Design review of the part built by this model. Coordinates are the model's own, in mm. A direction names the side the tool comes from. Coordinates: 2 decimals unless noted, no trailing zeros. Loops run counter-clockwise (first coordinate to the right, second up) from the corner with the lowest first, then second, coordinate; pieces in that order, holes last. Notation, with made-up numbers: (10.25, 37) -> (34.25, 37) arc R31 ccw to (34.25, 76) -> close; hole circle Ø1 at (26, 66.25). An arc over 180 degrees is marked (long way). One line per item, written item: value. Start each with the question number.
1. Add section B-B on y = -4. Write out the cut boundary in (x, z), plus the area to 3 significant figures.
2. Add section C-C on x = 0.25. Write out the cut boundary in (y, z).
3. Add section A-A on z = 5. Write out the cut boundary in (x, y), plus the area to 3 significant figures.
4. Insertion check: pin 1 (2 mm diameter, centred on x = -2, y = -12, fed in from -Z); pin 2 (2 mm diameter, centred on x = -18.5, y = -7.5, fed in from +Z); pin 3 (3 mm diameter, centred on x = -6.15, y = -8, fed in from +Z). Each pin has a flat end and moves straight along its axis. Give the tip position at first contact, or say it passes through.
5. Machinability: for faces 1 (the flat face through (-12, -8, -3.642)), 2 (the cylindrical face through (-4.49, -7.31, 0.8)), 3 (the cylindrical face through (-1.1, -10.3, 7.3)), which of the approach directions +Z, -Z, +X, -X, +Y, -Y give a long, thin tool a straight path to every point of the face, cutting with its end or side? Answer none if there is none.
6. For probe 1 along Y at (x, z) = (-6, 5); probe 2 along Y at (x, z) = (0, 4.25); probe 3 along Y at (x, z) = (-4, -1.25), list the stretches that pass through material, from the lowest coordinate up.
7. Draft analysis for pull direction Y (two halves, no side actions). For faces 4 (the flat face through (-13.47, -4.79, 1.61)), 5 (the flat face through (-2, -4, 8.358)), 6 (the flat face through (-8, 0, 0)), state which applies: pulls with the +Y half, pulls with the -Y half, needs draft (parallel to the pull), parting line crosses it, or undercut.
8. Add section D-D on y = -8. Write out the cut boundary in (x, z).
```python
from build123d import *

# Parameters (mm, degrees)
F1_DEPTH = 16
F2_R     = 2
F3_DEPTH = 2
F4_T     = -1
F5_R     = 2.8
F5_R_2   = 1.8


with BuildPart() as f1:
    # F0 (on Front) → F1 (new body)
    with BuildSketch(Plane.XZ):
        Polygon((-22.2741838526, -1.6455285968), (-22.1515364396, -3.6417644576), (1.8484635604, -3.6417644576), (1.8484635604, 6.3582355424), (-6.1515364396, 6.3582355424), align=None)
    extrude(amount=F1_DEPTH)

    # F2 (on face) → F3 (join)
    with BuildSketch(Plane.XY.offset(6.3582355424)):
        with Locations((-2.1515364396, -4)):
            Circle(F2_R)
        with Locations((-2.1515364396, -12)):
            Circle(F2_R)
    extrude(amount=F3_DEPTH)

    # F4
    f4_openings = [f1.faces().sort_by_distance(p)[0] for p in [
        (-10.151536, -8, -3.641764),
    ]]
    offset(amount=F4_T, openings=f4_openings, kind=Kind.INTERSECTION)

    # F5 (on face) → F6 (join, up to the next surface of F1)
    with BuildSketch(Plane(origin=(0, 0, -3.6417644576), x_dir=(1, 0, 0), z_dir=(0, 0, -1))):
        with Locations((-6.1515364396, 8.0000003978)):
            Circle(F5_R)
        with Locations((-6.1515364396, 8.0000003978)):
            Circle(F5_R_2, mode=Mode.SUBTRACT)
        with Locations((-14.1496508211, 8.0000003978)):
            Circle(F5_R)
        with Locations((-14.1496508211, 8.0000003978)):
            Circle(F5_R_2, mode=Mode.SUBTRACT)
    extrude(until=Until.NEXT, dir=(0, 0, 1))


solid = f1.part
```
Worked answers:
1. outline: (-22.27, -1.65) -> (-22.15, -3.64) -> (-21.15, -3.64) -> (-21.24, -2.25) -> (-5.92, 5.36) -> (-3.15, 5.36) -> (-3.15, 7.36) -> (-1.15, 7.36) -> (-1.15, 5.36) -> (0.85, 5.36) -> (0.85, -3.64) -> (1.85, -3.64) -> (1.85, 6.36) -> (-0.15, 6.36) -> (-0.15, 8.36) -> (-4.15, 8.36) -> (-4.15, 6.36) -> (-6.15, 6.36) -> close
1. area: 40.1 mm²
2. outline: (-16, -3.64) -> (-15, -3.64) -> (-15, 5.36) -> (-1, 5.36) -> (-1, -3.64) -> (0, -3.64) -> (0, 6.36) -> (-16, 6.36) -> close
3. outline: (-8.89, -16) -> (1.85, -16) -> (1.85, 0) -> (-8.89, 0) -> close; hole (-6.64, -15) -> (0.85, -15) -> (0.85, -1) -> (-6.64, -1) -> (-6.64, -5.24) arc R2.8 cw (long way) to (-6.64, -10.76) -> close; hole (-6.64, -9.73) arc R1.8 ccw (long way) to (-6.64, -6.27) -> close
3. area: 75.2 mm²
4. pin 1: stops at z = 5.36
4. pin 2: stops at z = 0.72
4. pin 3: stops at z = 6.36
5. face 1: -Z, +X, -X, +Y, -Y
5. face 2: -Z
5. face 3: +Z
6. probe 1: y = -16 to -15, -10.8 to -9.79, -6.21 to -5.2, -1 to 0
6. probe 2: y = -16 to -15, -1 to 0
6. probe 3: y = -16 to -15, -9.79 to -6.21, -1 to 0
7. face 4: undercut
7. face 5: needs draft
7. face 6: pulls with the +Y half
8. outline: (-22.27, -1.65) -> (-22.15, -3.64) -> (-21.15, -3.64) -> (-21.24, -2.25) -> (-16.95, -0.12) -> (-16.95, -3.64) -> (-15.95, -3.64) -> (-15.95, 0.38) -> (-12.35, 2.16) -> (-12.35, -3.64) -> (-11.35, -3.64) -> (-11.35, 2.66) -> (-8.95, 3.85) -> (-8.95, -3.64) -> (-7.95, -3.64) -> (-7.95, 4.35) -> (-5.92, 5.36) -> (-4.35, 5.36) -> (-4.35, -3.64) -> (-3.35, -3.64) -> (-3.35, 5.36) -> (0.85, 5.36) -> (0.85, -3.64) -> (1.85, -3.64) -> (1.85, 6.36) -> (-6.15, 6.36) -> close
